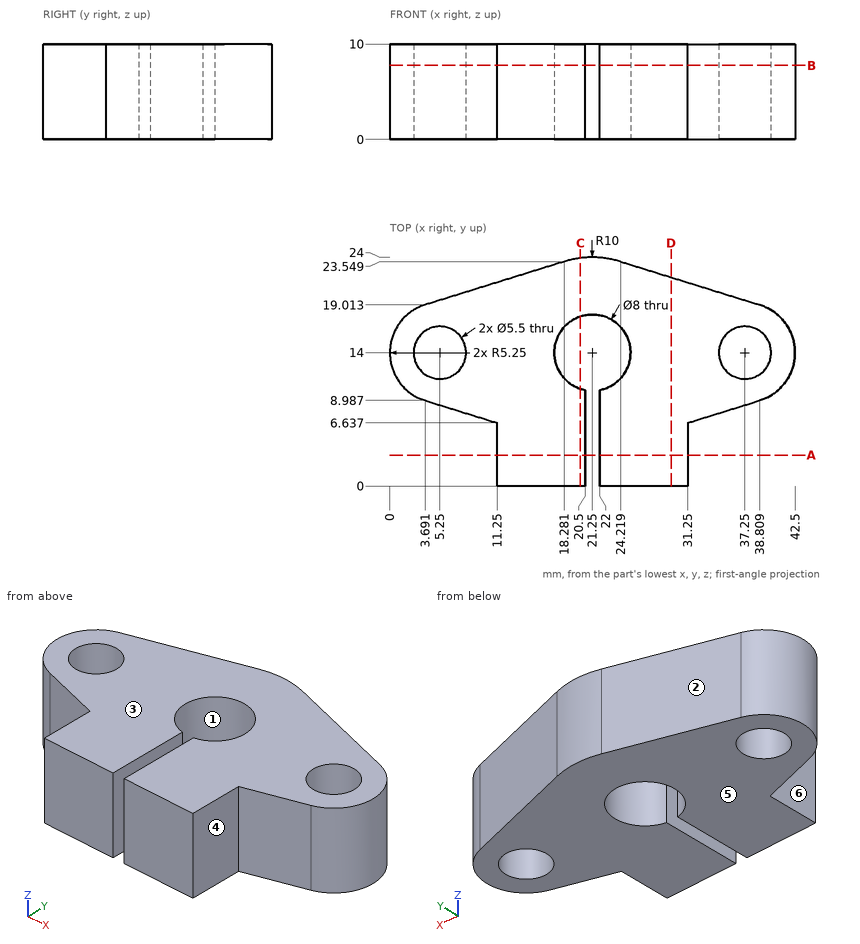
Answer from the drawing. Dimensions are ordinates in mm from the lowest x, y and z of the part. A direction names the side the tool comes from. Round coordinates to 2 decimals unless told otherwise and drop trailing zeros. Loops run counter-clockwise (first coordinate to the right, second up) from the corner with the lowest first, then second, coordinate; pieces in that order, holes last.
Q1. Each of these flat-tipped pins is pushed along its axis until it touches: pin 1 (3.5 mm diameter, centred on y = 3, z = 6.5, fed in from +X); pin 2 (3.5 mm diameter, centred on y = 3.5, z = 7.5, fed in from -X); pin 3 (1.5 mm diameter, centred on y = 11.5, z = 4.5, fed in from +X). Where does it stop, or does it pass through?
Q2. Section A-A on y = 3.25 is taken. Write down the section's boundary in (x, z).
Q3. Consider probe 1 along X at (y, z) = (12.25, 9.75) (1 decimal); probe 2 along X at (y, z) = (14.5, 3.5) (1 decimal); probe 3 along X at (y, z) = (2.75, 5.75). Determine where each line is inside the solid, lowest interval first.
Q4. Which of the six approach directions +Z, -Z, +X, -X, +Y, -Y give full straight-line access (tool end or side, diameter ignored) to the marked faces 5 and 6?
Q5. Section D-D on x = 29.5 is taken. Write down the section's boundary in (y, z), and give its area (3 significant figures).
Q6. Section C-C on x = 20 is taken. Write down the section's boundary in (y, z).
Q7. Determine the mould class of the marked faces 1, 2, 3 and 4 for opening direction X: released by +X, released by -X, zero draft, split by the parting line, or undercut.
Q8. Section B-B on z = 7.75 is taken. Write down the section's boundary in (x, y), and give its area (3 significant figures).
Output:
1. pin 1: stops at x = 31.25
1. pin 2: stops at x = 11.25
1. pin 3: stops at x = 42.2
2. outline: (11.25, 0) - (20.5, 0) - (20.5, 10) - (11.25, 10) - close; (22, 0) - (31.25, 0) - (31.25, 10) - (22, 10) - close
3. probe 1: x = 0.3 to 3.1, 7.4 to 17.7, 24.8 to 35.1, 39.4 to 42.2
3. probe 2: x = 0 to 2.5, 8 to 17.3, 25.2 to 34.5, 40 to 42.5
3. probe 3: x = 11.25 to 20.5, 22 to 31.25
4. face 5: -Z, +X, -X, +Y, -Y
4. face 6: +Z, -Z, -X, -Y
5. outline: (0, 0) - (21.91, 0) - (21.91, 10) - (0, 10) - close
5. area: 219 mm2
6. outline: (0, 0) - (10.2, 0) - (10.2, 10) - (0, 10) - close; (17.8, 0) - (23.92, 0) - (23.92, 10) - (17.8, 10) - close
7. face 1: undercut
7. face 2: released by -X
7. face 3: zero draft
7. face 4: released by +X
8. outline: (3.69, 8.99) - (11.25, 6.64) - (11.25, 0) - (20.5, 0) - (20.5, 10.07) arc R4 cw (long way) to (22, 10.07) - (22, 0) - (31.25, 0) - (31.25, 6.64) - (38.81, 8.99) arc R5.25 ccw to (38.81, 19.01) - (24.22, 23.55) arc R10 ccw to (18.28, 23.55) - (3.69, 19.01) arc R5.25 ccw to start; hole circle Ø5.5 at (5.25, 14); hole circle Ø5.5 at (37.25, 14)
8. area: 586 mm2
